```python
from build123d import *

# Parameters (mm, degrees)
SKETCH1_W           = 279.4
SKETCH1_H           = 304.8
BOSS_EXTRUDE1_DEPTH = 5
CUT_EXTRUDE1_DEPTH  = 10
SKETCH3_R           = 2.125
CUT_EXTRUDE2_DEPTH  = 198.169368818
SKETCH6_R           = 2
SKETCH6_R_2         = 31.1
CUT_EXTRUDE3_DEPTH  = 198.169368818
SKETCH5_R           = 1.5875
CUT_EXTRUDE4_DEPTH  = 10
FILLET1_R           = 10


with BuildPart() as part:
    # Sketch1 → Boss-Extrude1 (new body)
    with BuildSketch(Plane(origin=(0, 0, 0), x_dir=(1, 0, 0), z_dir=(0, 1, 0))):
        Rectangle(SKETCH1_W, SKETCH1_H)
    extrude(amount=BOSS_EXTRUDE1_DEPTH)

    # Sketch2 → Cut-Extrude1 (cut)
    with BuildSketch(Plane(origin=(0, 5, 0), x_dir=(1, 0, 0), z_dir=(0, 1, 0))):
        Polygon((-139.7, 152.4), (-85, 152.4), (-85, 117.4), (-125, 117.4), (-125, -117.4), (-85, -117.4), (-85, -152.4), (-139.7, -152.4), align=None)
        Polygon((139.7, -152.4), (85, -152.4), (85, -117.4), (125, -117.4), (125, 117.4), (85, 117.4), (85, 152.4), (139.7, 152.4), align=None)
    extrude(amount=-CUT_EXTRUDE1_DEPTH, mode=Mode.SUBTRACT)

    # Sketch3 → Cut-Extrude2 (cut, through all)
    with BuildSketch(Plane(origin=(0, 5, 0), x_dir=(1, 0, 0), z_dir=(0, 1, 0))):
        with Locations(Location((-75, 142.4, 0), (0, 0, 270))):
            Circle(SKETCH3_R)
        with Locations(Location((75, 142.4, 0), (0, 0, 270))):
            Circle(SKETCH3_R)
        with Locations(Location((75, -142.4, 0), (0, 0, 270))):
            Circle(SKETCH3_R)
        with Locations(Location((-75, -142.4, 0), (0, 0, 270))):
            Circle(SKETCH3_R)
        with Locations(Location((0, 142.4, 0), (0, 0, 270))):
            Circle(SKETCH3_R)
        with Locations(Location((0, -142.4, 0), (0, 0, 270))):
            Circle(SKETCH3_R)
    extrude(amount=-CUT_EXTRUDE2_DEPTH, mode=Mode.SUBTRACT)

    # Sketch6 → Cut-Extrude3 (cut, through all)
    with BuildSketch(Plane(origin=(0, 5, 0), x_dir=(1, 0, 0), z_dir=(0, 1, 0))):
        with Locations(Location((-110, 102.4, 0), (0, 0, 270))):
            Circle(SKETCH6_R)
        with Locations(Location((-47.8, 102.4, 0), (0, 0, 270))):
            Circle(SKETCH6_R)
        with Locations(Location((-47.8, 40.2, 0), (0, 0, 270))):
            Circle(SKETCH6_R)
        with Locations(Location((-110, 40.2, 0), (0, 0, 270))):
            Circle(SKETCH6_R)
        with Locations(Location((-110, -5.2, 0), (0, 0, 270))):
            Circle(SKETCH6_R)
        with Locations(Location((-47.8, -5.2, 0), (0, 0, 270))):
            Circle(SKETCH6_R)
        with Locations(Location((-47.8, -67.4, 0), (0, 0, 270))):
            Circle(SKETCH6_R)
        with Locations(Location((-110, -67.4, 0), (0, 0, 270))):
            Circle(SKETCH6_R)
        with Locations(Location((-78.9, 71.3, 0), (0, 0, 270))):
            Circle(SKETCH6_R_2)
        with Locations(Location((-78.9, -36.3, 0), (0, 0, 270))):
            Circle(SKETCH6_R_2)
        with Locations(Location((78.9, -36.3, 0), (0, 0, 90))):
            Circle(SKETCH6_R_2)
        with Locations(Location((78.9, 71.3, 0), (0, 0, 90))):
            Circle(SKETCH6_R_2)
        with Locations(Location((110, -67.4, 0), (0, 0, 90))):
            Circle(SKETCH6_R)
        with Locations(Location((47.8, -67.4, 0), (0, 0, 90))):
            Circle(SKETCH6_R)
        with Locations(Location((47.8, -5.2, 0), (0, 0, 90))):
            Circle(SKETCH6_R)
        with Locations(Location((110, -5.2, 0), (0, 0, 90))):
            Circle(SKETCH6_R)
        with Locations(Location((110, 40.2, 0), (0, 0, 90))):
            Circle(SKETCH6_R)
        with Locations(Location((47.8, 40.2, 0), (0, 0, 90))):
            Circle(SKETCH6_R)
        with Locations(Location((47.8, 102.4, 0), (0, 0, 90))):
            Circle(SKETCH6_R)
        with Locations(Location((110, 102.4, 0), (0, 0, 90))):
            Circle(SKETCH6_R)
    extrude(amount=-CUT_EXTRUDE3_DEPTH, mode=Mode.SUBTRACT)

    # Sketch5 → Cut-Extrude4 (cut)
    with BuildSketch(Plane(origin=(0, 5, 0), x_dir=(1, 0, 0), z_dir=(0, 1, 0))):
        with Locations(Location((24.120614372, 111.137541604, 0), (0, 0, 270))):
            Circle(SKETCH5_R)
        with Locations(Location((-24.139385628, 104.787541604, 0), (0, 0, 270))):
            Circle(SKETCH5_R)
        with Locations(Location((-8.899385628, 80.657541604, 0), (0, 0, 270))):
            Circle(SKETCH5_R)
        with Locations(Location((19.040614372, 80.657541604, 0), (0, 0, 270))):
            Circle(SKETCH5_R)
        with Locations(Location((24.120614372, 28.587541604, 0), (0, 0, 270))):
            Circle(SKETCH5_R)
        with Locations(Location((-24.139385628, 29.857541604, 0), (0, 0, 270))):
            Circle(SKETCH5_R)
        Polygon((0, 66.727836804), (-25, 66.727836804), (-25, 45.310060528), (-14.26649767, 45.310060528), (-14.26649767, 0), (-25, 0), (-25, -110), (25, -110), (25, 0), (15.644534715, 0), (15.644534715, 45.310060528), (25, 45.310060528), (25, 66.727836804), (11.213270658, 66.727836804), (11.213270658, 115.102469427), (0, 115.102469427), (-17.849370469, 115.102469427), (-17.849370469, 97.688471773), (0, 97.688471773), align=None)
    extrude(amount=-CUT_EXTRUDE4_DEPTH, mode=Mode.SUBTRACT)

    # Fillet1
    # the kernel refuses this fillet: 10 mm, written as the material it adds along each edge
    with BuildSketch(Plane(origin=(-85, 5, -117.4), x_dir=(0, 0, -1), z_dir=(0, -1, 0)), Plane(origin=(-85, 5, 117.4), x_dir=(-1, 0, 0), z_dir=(0, -1, 0)), Plane(origin=(-17.849370469, 5, -115.102469427), x_dir=(0, 0, 1), z_dir=(0, -1, 0)), Plane(origin=(11.213270658, 5, -115.102469427), x_dir=(-1, 0, 0), z_dir=(0, -1, 0)), Plane(origin=(25, 5, 110), x_dir=(0, 0, -1), z_dir=(0, -1, 0)), Plane(origin=(-25, 5, 110), x_dir=(1, 0, 0), z_dir=(0, -1, 0))) as fillet1_piece_1:
        with BuildLine():
            CenterArc((FILLET1_R, -FILLET1_R), FILLET1_R, 90, 90)
            Line((0, -FILLET1_R), (0, 0))
            Line((0, 0), (FILLET1_R, 0))
        make_face()
    extrude(amount=5)
    with BuildSketch(Plane(origin=(-25, 5, -66.727836804), x_dir=(1, 0, 0), z_dir=(0, -1, 0)), Plane(origin=(85, 5, 117.4), x_dir=(1, 0, 0), z_dir=(0, -1, 0)), Plane(origin=(85, 5, -117.4), x_dir=(0, 0, -1), z_dir=(0, -1, 0))) as fillet1_piece_2:
        with BuildLine():
            CenterArc((FILLET1_R, FILLET1_R), FILLET1_R, 180, 90)
            Line((0, FILLET1_R), (0, 0))
            Line((0, 0), (FILLET1_R, 0))
        make_face()
    extrude(amount=5)
    # the kernel refuses this fillet: 10 mm, written as the material it takes off along each edge
    with BuildSketch(Plane(origin=(-85, 30, -152.4), x_dir=(1, 0, 0), z_dir=(0, -1, 0)), Plane(origin=(-125, 30, -117.4), x_dir=(1, 0, 0), z_dir=(0, -1, 0)), Plane(origin=(-125, 30, 117.4), x_dir=(0, 0, -1), z_dir=(0, -1, 0)), Plane(origin=(-85, 30, 152.4), x_dir=(0, 0, -1), z_dir=(0, -1, 0)), Plane(origin=(-14.26649767, 30, 0), x_dir=(-1, 0, 0), z_dir=(0, -1, 0)), Plane(origin=(-14.26649767, 30, -45.310060528), x_dir=(0, 0, 1), z_dir=(0, -1, 0)), Plane(origin=(0, 30, -66.727836804), x_dir=(-1, 0, 0), z_dir=(0, -1, 0)), Plane(origin=(0, 30, -97.688471773), x_dir=(0, 0, 1), z_dir=(0, -1, 0)), Plane(origin=(11.213270658, 30, -66.727836804), x_dir=(0, 0, -1), z_dir=(0, -1, 0)), Plane(origin=(85, 30, 152.4), x_dir=(-1, 0, 0), z_dir=(0, -1, 0))) as fillet1_2_piece_1:
        with BuildLine():
            CenterArc((FILLET1_R, FILLET1_R), FILLET1_R, 180, 90)
            Line((0, FILLET1_R), (0, 0))
            Line((0, 0), (FILLET1_R, 0))
        make_face()
    extrude(amount=55, mode=Mode.SUBTRACT)
    with BuildSketch(Plane(origin=(15.644534715, 29.948017832, -45.310060528), x_dir=(1, 0, 0), z_dir=(0, -1, 0))) as fillet1_2_piece_2:
        with BuildLine():
            CenterArc((10, 9.979207133), FILLET1_R, 180, 86.304526435)
            Line((0, 9.979207133), (0, 0))
            Line((0, 0), (9.355465285, 0))
        make_face()
    extrude(amount=54.896035664, mode=Mode.SUBTRACT)
    with BuildSketch(Plane(origin=(15.644534715, 29.948017832, 0), x_dir=(0, 0, -1), z_dir=(0, -1, 0))) as fillet1_2_piece_3:
        with BuildLine():
            CenterArc((9.979207133, 10), FILLET1_R, 183.695473565, 86.304526435)
            Line((0, 9.355465285), (0, 0))
            Line((0, 0), (9.979207133, 0))
        make_face()
    extrude(amount=54.896035664, mode=Mode.SUBTRACT)
    with BuildSketch(Plane(origin=(125, 30, 117.4), x_dir=(0, 0, -1), z_dir=(0, -1, 0)), Plane(origin=(125, 30, -117.4), x_dir=(-1, 0, 0), z_dir=(0, -1, 0)), Plane(origin=(85, 30, -152.4), x_dir=(-1, 0, 0), z_dir=(0, -1, 0))) as fillet1_2_piece_4:
        with BuildLine():
            CenterArc((FILLET1_R, -FILLET1_R), FILLET1_R, 90, 90)
            Line((0, -FILLET1_R), (0, 0))
            Line((0, 0), (FILLET1_R, 0))
        make_face()
    extrude(amount=55, mode=Mode.SUBTRACT)


solid = part.part
```
Geometry: final body of the model. Coordinates: model frame, mm. A direction names the side the tool comes from. Give positions to 0.01 mm unless a question says otherwise; leave off trailing zeros. Write each loop counter-clockwise with the first axis right and the second up, starting at its lowest first coordinate (ties: lowest second). Pieces come first, ordered by that corner, then holes.
1. Reachability of faces 1 (the cylindrical face through (-87.85, 2.54, -120.41)), 2 (the cylindrical face through (14.2, 2.5, -69.6)) from +Z, -Z, +X, -X, +Y, -Y: full face, straight path, thin tool, end or side. Return the list, or none.
2. Section query B-B, the plane x = -104. Return loops of the section in (y, z).
3. Section query D-D, the plane x = -64. Return loops of the section in (y, z), then the cut area to 3 significant figures.
4. Line query: probe 1 along X at (y, z) = (1.15, 142.4) (3 decimals); probe 2 along Z at (x, y) = (-111, 2.6); probe 3 along X at (y, z) = (0.95, 36). Output: solid intervals per line, ascending.
5. Pin query (flat end, axial travel): P1, Ø3, axis at x = -47.8, z = -102.4, coming from the +Y side; P2, Ø3, axis at x = 77, y = 2.5, coming from the +Z side; P3, Ø4.5, axis at x = 47.8, z = -40.2, coming from the +Y side; P4, Ø1.5, axis at y = 1.5, z = -131.5, coming from the -X side. Return the tip coordinate at first contact, or that it passes through.
6. Section query C-C, the plane z = 36. Return loops of the section in (x, y), then the cut area to 3 significant figures.
7. Section query A-A, the plane z = -71.3. Return loops of the section in (x, y), then the cut area to 3 significant figures.
8. Draft query along X for faces 3 (the cylindrical face through (-2.852, 2.535, -69.735)), 4 (the cylindrical face through (88.01, 2.54, -120.25)), 5 (the flat face through (30, 5, 2)). Return one class per face: released by +X, released by -X, zero draft, split by the parting line, or undercut.
Computed:
1. face 1: -Z, -X, +Y, -Y
1. face 2: +Y, -Y
2. outline: (0, -117.4) - (5, -117.4) - (5, -89.66) - (0, -89.66) - close; (0, -52.94) - (5, -52.94) - (5, 17.94) - (0, 17.94) - close; (0, 54.66) - (5, 54.66) - (5, 117.4) - (0, 117.4) - close
3. outline: (0, -152.4) - (5, -152.4) - (5, -98.6) - (0, -98.6) - close; (0, -44) - (5, -44) - (5, 9) - (0, 9) - close; (0, 63.6) - (5, 63.6) - (5, 152.4) - (0, 152.4) - close
3. area: 978 mm2
4. probe 1: x = -85 to -77.125, -72.875 to -2.125, 2.125 to 72.875, 77.125 to 85
4. probe 2: z = -117.4 to -104.13, -100.67 to -41.93, -38.47 to 3.47, 6.93 to 65.67, 69.13 to 117.4
4. probe 3: x = -125 to -110, -47.8 to -25, 25 to 47.8, 110 to 125
5. P1: passes through
5. P2: stops at z = 152.39
5. P3: stops at y = 5
5. P4: stops at x = -85
6. outline: (-125, 0) - (-110, 0) - (-110, 5) - (-125, 5) - close; (-47.8, 0) - (-25, 0) - (-25, 5) - (-47.8, 5) - close; (25, 0) - (47.8, 0) - (47.8, 5) - (25, 5) - close; (110, 0) - (125, 0) - (125, 5) - (110, 5) - close
6. area: 378 mm2
7. outline: (-125, 0) - (-110, 0) - (-110, 5) - (-125, 5) - close; (-47.8, 0) - (-1.6, 0) - (-1.6, 5) - (-47.8, 5) - close; (12.81, 0) - (47.8, 0) - (47.8, 5) - (12.81, 5) - close; (110, 0) - (125, 0) - (125, 5) - (110, 5) - close
7. area: 556 mm2
8. face 3: undercut
8. face 4: released by +X
8. face 5: zero draft
